```python
from build123d import *

# Parameters (mm, degrees)
F0_W     = 19.05
F0_H     = 723.9
F1_DEPTH = 76.2


with BuildPart() as f1:
    # F0 (on Top) → F1 (new body)
    with BuildSketch(Plane.XY):
        Polygon((762, 381), (-762, 381), (-762, 361.95), (-742.95, 361.95), (742.95, 361.95), (762, 361.95), align=None)
        with Locations((-752.475, 0)):
            Rectangle(F0_W, F0_H)
        Polygon((-742.95, -361.95), (-762, -361.95), (-762, -381), (762, -381), (762, -361.95), (742.95, -361.95), align=None)
        with Locations((752.475, 0)):
            Rectangle(F0_W, F0_H)
    extrude(amount=F1_DEPTH)


solid = f1.part
```
Here's how the part is built. I have some questions about the finished solid (model axes, mm). A direction names the side the tool comes from. Coordinates: 2 decimals unless noted, no trailing zeros. Write each loop counter-clockwise with the first axis right and the second up, starting at its lowest first coordinate (ties: lowest second). Pieces come first, ordered by that corner, then holes. Notation, with made-up numbers: M -1,44.5 L 32,44.5 A18 cw 32,67.5 Z; hole C 35,25.5 d3. An arc over 180 degrees is marked long. Answer as CSV lines item,"result". Start each with the question number.
Q1. If we mould it in two halves opening along Y, with no side actions, what happens to faces 3 (the flat face through (-742.95, -5, 38)), 4 (the flat face through (-4, 369, 76.2)), 5 (the flat face through (-11, -381, 38)), 6 (the flat face through (11, 381, 38))? For each: pulls with the +Y half, pulls with the -Y half, needs draft (parallel to the pull), parting line crosses it, or undercut.
Q2. I need wall thicknesses on probe 1 along X at (y, z) = (145, 52); probe 2 along Y at (x, z) = (440.5, 52.5). Which ranges of each line are inside material? Lowest first, please. Write a range as [from, to].
Q3. Suppose I cut it at A-A, the plane x = 309. List the corners of the cut face in (y, z) for me, then the cut area to 3 significant figures.
Q4. For faces 1 (the flat face through (742.95, -5, 38)), 2 (the flat face through (-762, 5, 38)), which set-ups out of +Z, -Z, +X, -X, +Y, -Y let a thin tool reach every point of the face, with its end or its side?
Q5. Suppose I cut it at C-C, the plane z = 20. List the corners of the cut face in (x, y) for me.
Q6. Suppose I cut it at B-B, the plane y = 130.5. List the corners of the cut face in (x, z) for me, then the cut area to 3 significant figures.
Entries:
1,face 3,"undercut"
1,face 4,"needs draft"
1,face 5,"pulls with the -Y half"
1,face 6,"pulls with the +Y half"
2,probe 1,"x = [-762, -742.95], [742.95, 762]"
2,probe 2,"y = [-381, -361.95], [361.95, 381]"
3,outline,"M -381,0 L -361.95,0 L -361.95,76.2 L -381,76.2 Z; M 361.95,0 L 381,0 L 381,76.2 L 361.95,76.2 Z"
3,area,"2,900 mm²"
4,face 1,"+Z, -Z"
4,face 2,"+Z, -Z, -X, +Y, -Y"
5,outline,"M -762,-381 L 762,-381 L 762,381 L -762,381 Z; hole M -742.95,-361.95 L 742.95,-361.95 L 742.95,361.95 L -742.95,361.95 Z"
6,outline,"M -762,0 L -742.95,0 L -742.95,76.2 L -762,76.2 Z; M 742.95,0 L 762,0 L 762,76.2 L 742.95,76.2 Z"
6,area,"2,900 mm²"
